The listing builds one solid part. Answer for the finished solid, in the listing's coordinates (mm). A direction names the side the tool comes from. Round coordinates to 2 decimals unless told otherwise and drop trailing zeros. Order: outer loops, then holes, each group sorted by start corner. A loop starts at its lowest first (then second) coordinate and runs counter-clockwise, first axis right, second up. Notation, with made-up numbers: M -5,-33 L 25,-33 A16 ccw 25,-4 Z; hole C 25.25,72 d11. An arc over 180 degrees is marked long. Write item = value, one per line. Start each with the question number.
(1) A cutting plane is placed at C-C, the plane y = 1.6. Determine the outline of the cut face in (x, z).
(2) Straight lines are drawn through the part: probe 1 along X at (y, z) = (0.6, -49); probe 2 along Z at (x, y) = (125, 1.65); probe 3 along Z at (x, y) = (119.3, 1.8). For each, find the intervals that lie inside material, in ascending order. Write a range as from..to.
(3) Each of these flat-tipped pins is pushed along its axis until it touches: pin 1 (0.8 mm diameter, centred on x = 144.5, y = 1, fed in from +Z); pin 2 (1.4 mm diameter, centred on x = -6.5, y = 2, fed in from -Z); pin 3 (1.4 mm diameter, centred on y = 1.5, z = -64.5, fed in from -X). Where does it stop, or does it pass through?
(4) A cutting plane is placed at D-D, the plane z = -21. Determine the outline of the cut face in (x, y).
(5) A cutting plane is placed at A-A, the plane x = 119.3. Determine the outline of the cut face in (y, z).
(6) Which of the six approach directions +Z, -Z, +X, -X, +Y, -Y give full straight-line access (tool end or side, diameter ignored) to faces 1 (the face through (129, 1, -63)), 2 (the face through (79, 1, -63)), 3 (the face through (145, 1, -18.567)), 4 (the face through (71, 2.7, -31)), 5 (the face through (-6, 1, -42.133))?
(7) A cutting plane is placed at B-B, the plane z = -49. Determine the outline of the cut face in (x, y).
from build123d import *

# Parameters (mm, degrees)
SKETCH1_R           = 1.75
BOSS_EXTRUDE1_DEPTH = 2.7


with BuildPart() as part:
    # Sketch1 → Boss-Extrude1 (new body)
    with BuildSketch(Plane(origin=(0, 0, 0), x_dir=(1, 0, 0), z_dir=(0, 1, 0))):
        Polygon((64.5, 63), (64.5, 58), (74.5, 58), (74.5, 63), (84.4, 63), (84.4, 65.7), (114.2, 65.7), (114.2, 63), (144, 63), (144, 42.133333333), (146.7, 42.133333333), (146.7, 18.566666667), (144, 18.566666667), (144, -5), (115.82, -5), (84.94, -5), (74.5, -5), (64.5, -5), (54.06, -5), (23.18, -5), (-5, -5), (-5, 18.566666667), (-7.7, 18.566666667), (-7.7, 42.133333333), (-5, 42.133333333), (-5, 63), (24.8, 63), (24.8, 65.7), (54.6, 65.7), (54.6, 63), align=None)
        with Locations((13.3, 21)):
            Circle(SKETCH1_R, mode=Mode.SUBTRACT)
        with Locations((14.3, 49)):
            Circle(SKETCH1_R, mode=Mode.SUBTRACT)
        with Locations((119.3, 49)):
            Circle(SKETCH1_R, mode=Mode.SUBTRACT)
        with Locations((125, 21)):
            Circle(SKETCH1_R, mode=Mode.SUBTRACT)
    extrude(amount=BOSS_EXTRUDE1_DEPTH)


solid = part.part
Reported:
q1.outline = M -7.7,-42.13 L -5,-42.13 L -5,-63 L 24.8,-63 L 24.8,-65.7 L 54.6,-65.7 L 54.6,-63 L 64.5,-63 L 64.5,-58 L 74.5,-58 L 74.5,-63 L 84.4,-63 L 84.4,-65.7 L 114.2,-65.7 L 114.2,-63 L 144,-63 L 144,-42.13 L 146.7,-42.13 L 146.7,-18.57 L 144,-18.57 L 144,5 L -5,5 L -5,-18.57 L -7.7,-18.57 Z; hole C 13.3,-21 d3.5; hole C 14.3,-49 d3.5; hole C 119.3,-49 d3.5; hole C 125,-21 d3.5
q2.probe_1 = -5..12.55, 16.05..117.55, 121.05..144
q2.probe_2 = -63..-22.75, -19.25..5
q2.probe_3 = -63..-50.75, -47.25..5
q3.pin_1 = -18.57
q3.pin_2 = -42.13
q3.pin_3 = 24.8
q4.outline = M -7.7,0 L 11.55,0 L 11.55,2.7 L -7.7,2.7 Z; M 15.05,0 L 123.25,0 L 123.25,2.7 L 15.05,2.7 Z; M 126.75,0 L 146.7,0 L 146.7,2.7 L 126.75,2.7 Z
q5.outline = M 0,-63 L 2.7,-63 L 2.7,-50.75 L 0,-50.75 Z; M 0,-47.25 L 2.7,-47.25 L 2.7,5 L 0,5 Z
q6.face_1 = -Z, +X, +Y, -Y
q6.face_2 = -Z, +Y, -Y
q6.face_3 = +Z, +X, +Y, -Y
q6.face_4 = +Z, -Z, +X, -X, +Y
q6.face_5 = -Z, -X, +Y, -Y
q7.outline = M -5,0 L 12.55,0 L 12.55,2.7 L -5,2.7 Z; M 16.05,0 L 117.55,0 L 117.55,2.7 L 16.05,2.7 Z; M 121.05,0 L 144,0 L 144,2.7 L 121.05,2.7 Z
